For this review, take the finished solid that the model builds, in its own axes (mm). A direction names the side the tool comes from. Give positions to 0.01 mm unless a question says otherwise; leave off trailing zeros. Loops run counter-clockwise (first coordinate to the right, second up) from the corner with the lowest first, then second, coordinate; pieces in that order, holes last. Notation, with made-up numbers: (22.25, 12.25) -> (71.25, 12.25) arc R3 cw to (71.25, 16.25) -> close; hole circle Ø10 at (71.5, 16). An arc over 180 degrees is marked (long way). Write each question's results on one line, items separated by ' | '. Start each with the question number.
```python
from build123d import *
from build123d.topology import SkipClean

# Parameters (mm, degrees)
EXTRUDE_1_DEPTH     = 50
SKETCH_7_R          = 3
EXTRUDE_2_DEPTH     = 7
SKETCH_8_R          = 17
EXTRUDE_3_DEPTH     = 27
SKETCH_9_R          = 8
CUT_EXTRUDE_1_DEPTH = 3
SKETCH_11_W         = 12
SKETCH_11_H         = 11
CUT_EXTRUDE_3_DEPTH = 20
SKETCH_12_R         = 12
CUT_EXTRUDE_4_DEPTH = 21
SKETCH_13_R         = 7
CUT_EXTRUDE_5_DEPTH = 62.684682178


with BuildPart() as part:
    # Sketch 1 → Extrude 1 (new body)
    with BuildSketch(Plane.XY.offset(25)):
        with BuildLine():
            Line((-12, 0), (-7, 0))
            ThreePointArc((-7, 0), (0, 7), (7, 0))
            Line((7, 0), (12, 0))
            ThreePointArc((12, 0), (0, 12), (-12, 0))
        make_face()
    extrude(amount=-EXTRUDE_1_DEPTH)

    # Sketch 7 → Extrude 2 (add)
    with BuildSketch(Plane(origin=(0, 0, 0), x_dir=(1, 0, 0), z_dir=(0, 1, 0))):
        with BuildLine():
            Line((-17, -21), (17, -21))
            ThreePointArc((17, -21), (21.949747468, -18.949747468), (24, -14))
            Line((24, -14), (24, 14))
            ThreePointArc((24, 14), (21.949747468, 18.949747468), (17, 21))
            Line((17, 21), (-17, 21))
            ThreePointArc((-17, 21), (-21.949747468, 18.949747468), (-24, 14))
            Line((-24, 14), (-24, -14))
            ThreePointArc((-24, -14), (-21.949747468, -18.949747468), (-17, -21))
        make_face()
        with Locations(Location((-17, 14, 0), (0, 0, 270))):
            Circle(SKETCH_7_R, mode=Mode.SUBTRACT)
        with Locations(Location((17, 14, 0), (0, 0, 270))):
            Circle(SKETCH_7_R, mode=Mode.SUBTRACT)
        with Locations(Location((17, -14, 0), (0, 0, 270))):
            Circle(SKETCH_7_R, mode=Mode.SUBTRACT)
        with Locations(Location((-17, -14, 0), (0, 0, 270))):
            Circle(SKETCH_7_R, mode=Mode.SUBTRACT)
    extrude(amount=EXTRUDE_2_DEPTH)

    # Sketch 8 → Extrude 3 (add)
    with BuildSketch(Plane(origin=(0, 0, 0), x_dir=(1, 0, 0), z_dir=(0, 1, 0))):
        with Locations(Location((0, 0, 0), (0, 0, 55.016476916))):
            Circle(SKETCH_8_R)
    extrude(amount=EXTRUDE_3_DEPTH)

    # Sketch 9 → Cut-Extrude 1 (cut)
    with BuildSketch(Plane(origin=(0, 27, 0), x_dir=(1, 0, 0), z_dir=(0, 1, 0))):
        with Locations(Location((0, 0, 0), (0, 0, 270))):
            Circle(SKETCH_9_R)
    extrude(amount=-CUT_EXTRUDE_1_DEPTH, mode=Mode.SUBTRACT)

    # Sketch 11 → Cut-Extrude 3 (cut, symmetric)
    with BuildSketch(Plane.XY):
        with Locations((0, 21.5)):
            Rectangle(SKETCH_11_W, SKETCH_11_H)
    extrude(amount=CUT_EXTRUDE_3_DEPTH, both=True, mode=Mode.SUBTRACT)

    # Sketch 12 → Cut-Extrude 4 (cut)
    with BuildSketch(Plane(origin=(0, 0, 0), x_dir=(1, 0, 0), z_dir=(0, 1, 0))):
        with Locations(Location((0, 0, 0), (0, 0, 120))):
            Circle(SKETCH_12_R)
    extrude(amount=CUT_EXTRUDE_4_DEPTH, mode=Mode.SUBTRACT)

    # Sketch 13 → Cut-Extrude 5 (cut, through all)
    with SkipClean():  # the faces are left unmerged after this step: merging them gives an invalid solid
        with BuildSketch(Plane.XY.offset(25)):
            Circle(SKETCH_13_R)
        extrude(amount=-CUT_EXTRUDE_5_DEPTH, mode=Mode.SUBTRACT)
    add(part.part.scale(1), mode=Mode.REPLACE)  # the faces are merged on a copy


solid = part.part
```
1. We need section B-B (y = 2.25). Write out the cut boundary in (x, z).
2. We need section D-D (y = 19.25). Write out the cut boundary in (x, z), plus the area to 3 significant figures.
3. Draft analysis for pull direction X (two halves, no side actions). For faces 6 (the cylindrical face through (0, 12, -21)), 7 (the flat face through (-0.2, 7.4, 25)), 8 (the cylindrical face through (22, 3.5, -18.9)), 9 (the flat face through (9, 21, 1)), state which applies: released by +X, released by -X, zero draft, split by the parting line, or undercut.
4. Wall thickness on L1, parallel to X at y = 11.25, z = 0; L2, parallel to X at y = 4.5, z = -16; L3, parallel to X at y = 2.75, z = 0: over which ranges is each line inside the solid? List them lowest first.
5. We need section C-C (x = 0). Write out the cut boundary in (y, z).
6. For pin 1 Ø1.5 at (y, z) = (11, 3.5) entering from -X; pin 2 Ø6 at (x, y) = (0.5, 15.5) entering from +Z; pin 3 Ø8 at (y, z) = (15, 3.5) entering from -X; pin 4 Ø3.5 at (x, z) = (17, -14) entering from +Y, all flat-tipped, find the tip position at first contact; note any pin that passes through.
7. Machinability: for faces 1 (the cylindrical face through (0, 12, 21)), 2 (the flat face through (14, 3, -21)), 3 (the flat face through (-14, 3, -21)), 4 (the flat face through (7, 24, 0)), 5 (the flat face through (0, 16, 14)), which of the approach directions +Z, -Z, +X, -X, +Y, -Y give a long, thin tool a straight path to every point of the face, cutting with its end or side? Answer none if there is none.
8. We need section A-A (z = 0). Write out the cut boundary in (x, y).
Response:
1) outline: (-24, -14) arc R7 ccw to (-17, -21) -> (-11.79, -21) -> (-11.79, -25) -> (-6.63, -25) -> (-6.63, -10) arc R12 cw to (-6.63, 10) -> (-6.63, 25) -> (-11.79, 25) -> (-11.79, 21) -> (-17, 21) arc R7 ccw to (-24, 14) -> close; (6.63, -25) -> (11.79, -25) -> (11.79, -21) -> (17, -21) arc R7 ccw to (24, -14) -> (24, 14) arc R7 ccw to (17, 21) -> (11.79, 21) -> (11.79, 25) -> (6.63, 25) -> (6.63, 10) arc R12 cw to (6.63, -10) -> close; hole circle Ø6 at (-17, -14); hole circle Ø6 at (-17, 14); hole circle Ø6 at (17, -14); hole circle Ø6 at (17, 14)
2) outline: (-6, -15.91) -> (-6, -10.39) arc R12 cw to (-6, 10.39) -> (-6, 15.91) arc R17 ccw to start; (6, -15.91) arc R17 ccw to (6, 15.91) -> (6, 10.39) arc R12 cw to (6, -10.39) -> close | area: 332 mm2
3) face 6: split by the parting line | face 7: zero draft | face 8: released by +X | face 9: undercut
4) L1: x = -17 to -12, 12 to 17 | L2: x = -23.71 to -19.24, -14.76 to -5.36, 5.36 to 14.76, 19.24 to 23.71 | L3: x = -24 to -12, 12 to 24
5) outline: (7, -25) -> (12, -25) -> (12, -17) -> (16, -17) -> (16, -12) -> (7, -12) -> close; (7, 12) -> (16, 12) -> (16, 17) -> (12, 17) -> (12, 25) -> (7, 25) -> close
6) pin 1: stops at x = -16.78 | pin 2: stops at z = 17 | pin 3: stops at x = -17 | pin 4: passes through
7) face 1: +Z, +Y | face 2: -Z, +X, +Y | face 3: -Z, -X, +Y | face 4: +Y | face 5: +Z, -Z, +Y
8) outline: (-24, 0) -> (-12, 0) -> (-12, 21) -> (-6, 21) -> (-6, 24) -> (-8, 24) -> (-8, 27) -> (-17, 27) -> (-17, 7) -> (-24, 7) -> close; (6, 21) -> (12, 21) -> (12, 0) -> (24, 0) -> (24, 7) -> (17, 7) -> (17, 27) -> (8, 27) -> (8, 24) -> (6, 24) -> close
